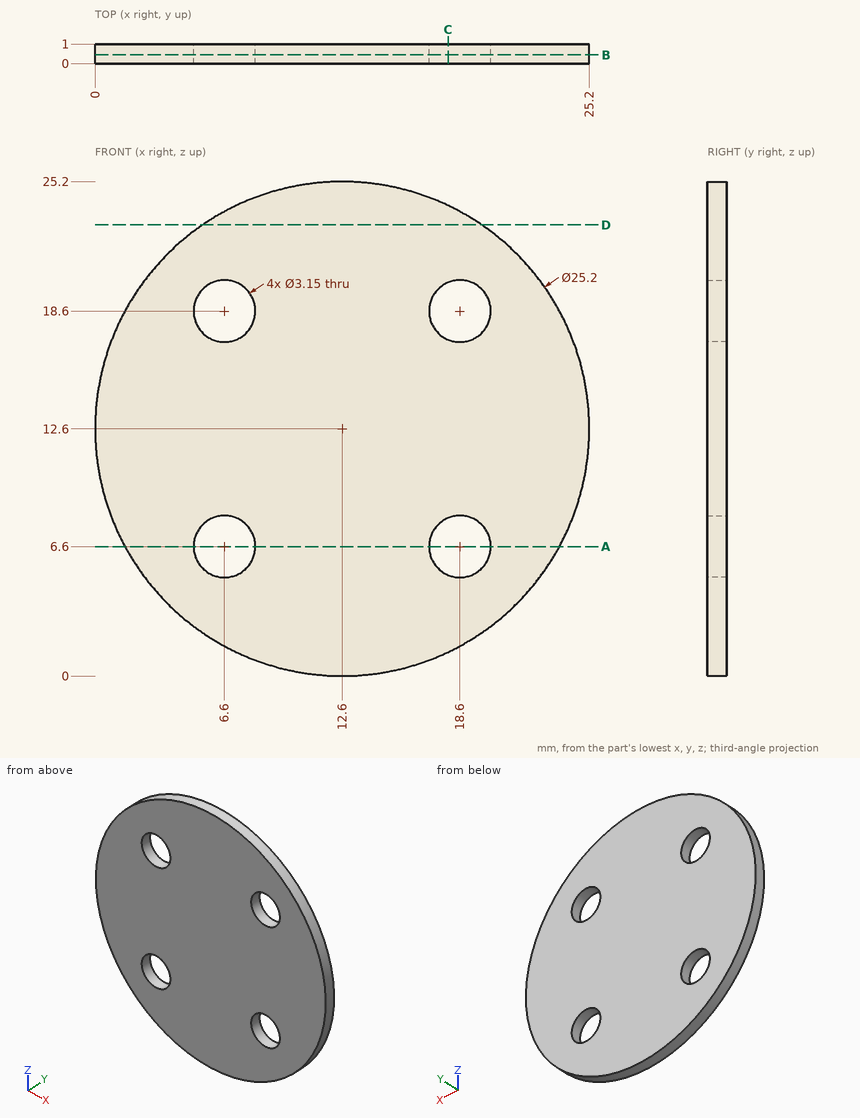
Design review of the part shown in the three views and the two pictorial views. Dimensions are in mm from the part's minimum x, y and z. Round coordinates to 2 decimals unless told otherwise and drop trailing zeros. Loops run counter-clockwise (first coordinate to the right, second up) from the corner with the lowest first, then second, coordinate; pieces in that order, holes last.
1) Consider section B-B on y = 0.45. State the section outline as (x, z) points (3 decimals), then the cut area to 3 significant figures.
Values follow:
outline: circle Ø25.2 at (12.6, 12.6); hole circle Ø3.15 at (6.6, 6.6); hole circle Ø3.15 at (6.6, 18.6); hole circle Ø3.15 at (18.6, 6.6); hole circle Ø3.15 at (18.6, 18.6)
area: 468 mm2
2) Consider section C-C on x = 18. State the section outline as (y, z) points, then the cut area to 3 significant figures.
Values follow:
outline: (0, 1.22) - (1, 1.22) - (1, 5.14) - (0, 5.14) - close; (0, 8.06) - (1, 8.06) - (1, 17.14) - (0, 17.14) - close; (0, 20.06) - (1, 20.06) - (1, 23.98) - (0, 23.98) - close
area: 16.9 mm2
3) Consider section A-A on z = 6.6. State the section outline as (x, y) points (3 decimals).
Values follow:
outline: (1.52, 0) - (5.025, 0) - (5.025, 1) - (1.52, 1) - close; (8.175, 0) - (17.025, 0) - (17.025, 1) - (8.175, 1) - close; (20.175, 0) - (23.68, 0) - (23.68, 1) - (20.175, 1) - close
4) Consider section D-D on z = 23. State the section outline as (x, y) points, then the cut area to 3 significant figures.
Values follow:
outline: (5.49, 0) - (19.71, 0) - (19.71, 1) - (5.49, 1) - close
area: 14.2 mm2
5) Wall thickness on line 1 along X through (y, z) = (0.7, 6.6) (3 decimals); line 2 along X through (y, z) = (0.6, 5.5): over which ranges is each line inside the solid? List them lowest first.
Values follow:
line 1: x = 1.52 to 5.025, 8.175 to 17.025, 20.175 to 23.68
line 2: x = 2.19 to 5.47, 7.73 to 17.47, 19.73 to 23.01
